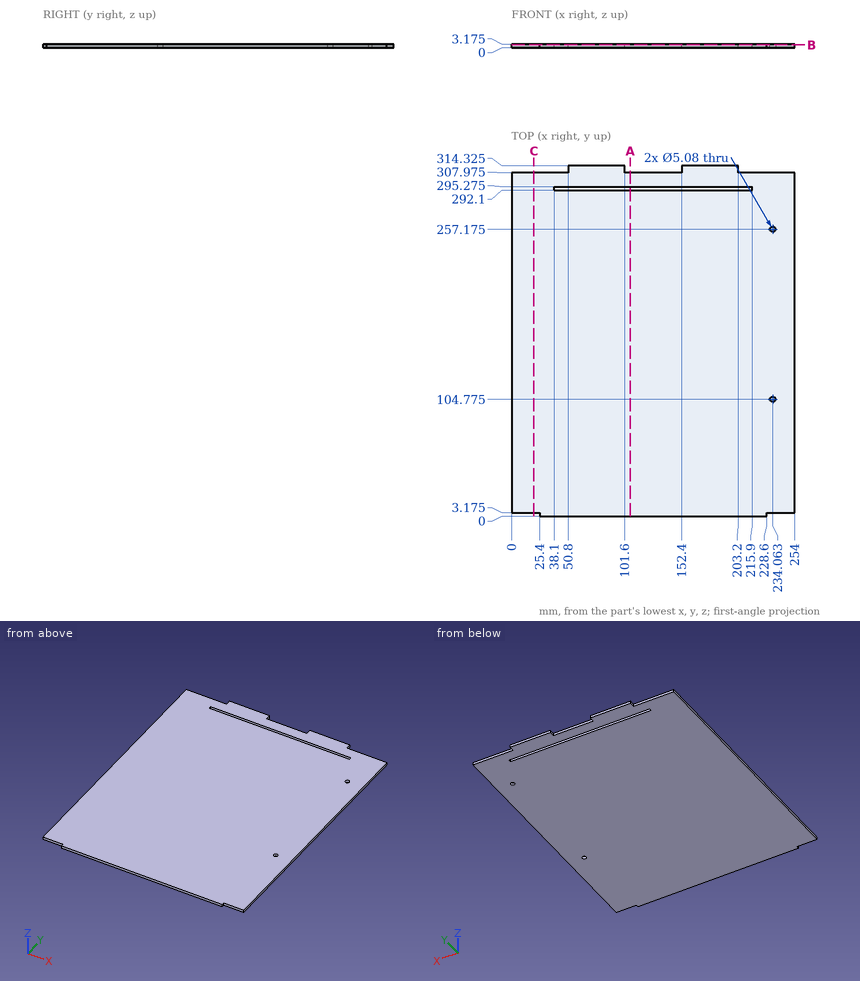
Verification items for this drawing (mm, ordinates from the low corner). Round coordinates to 2 decimals unless told otherwise and drop trailing zeros. Write each loop counter-clockwise with the first axis right and the second up, starting at its lowest first coordinate (ties: lowest second). Pieces come first, ordered by that corner, then holes. Notation, with made-up numbers: (-5.5, 83.5) - (30.5, 83.5) arc R35 cw to (30.5, 116.5) - close; hole circle Ø3 at (8, -10.5). An arc over 180 degrees is marked (long way). Answer as a JSON object with one key per item and string values. Group by question number.
Q1. Go/stop test with flat-tipped pins: pin 1 Ø1 at (y, z) = (294, 1.5) entering from -X; pin 2 Ø4.5 at (x, y) = (234.06, 104.78) entering from -Z; pin 3 Ø1.6 at (y, z) = (310, 1.5) entering from +X; pin 4 Ø1.6 at (x, z) = (246.5, 1.5) entering from -Y (3 decimals). Record where each tip stops, or that it passes through.
Q2. Section check C-C, the plane x = 20. Enter the section's corners in (y, z) (1 decimal).
Q3. Thickness scan on line 1 (Y direction, x = 174.5, z = 1.35) (1 decimal); line 2 (Y direction, x = 102, z = 1.7) (1 decimal); line 3 (Y direction, x = 221.5, z = 0.15) (1 decimal). Record the ranges inside material, lowest first.
Q4. Section check B-B, the plane z = 2.4. Enter the section's corners in (x, y) (1 decimal).
Q5. Section check A-A, the plane x = 106.5. Enter the section's corners in (y, z) (1 decimal).
Found:
{
 "1": {"pin 1": "stops at x = 0", "pin 2": "passes through", "pin 3": "stops at x = 203.2", "pin 4": "stops at y = 3.175"},
 "2": {"outline": "(3.2, 0) - (308, 0) - (308, 3.2) - (3.2, 3.2) - close"},
 "3": {"line 1": "y = 0 to 292.1, 295.3 to 314.3", "line 2": "y = 0 to 292.1, 295.3 to 308", "line 3": "y = 0 to 308"},
 "4": {"outline": "(0, 3.2) - (25.4, 3.2) - (25.4, 0) - (228.6, 0) - (228.6, 3.2) - (254, 3.2) - (254, 308) - (203.2, 308) - (203.2, 314.3) - (152.4, 314.3) - (152.4, 308) - (101.6, 308) - (101.6, 314.3) - (50.8, 314.3) - (50.8, 308) - (0, 308) - close; hole (38.1, 292.1) - (215.9, 292.1) - (215.9, 295.3) - (38.1, 295.3) - close; hole circle Ø5.1 at (234.1, 104.8); hole circle Ø5.1 at (234.1, 257.2)"},
 "5": {"outline": "(0, 0) - (292.1, 0) - (292.1, 3.2) - (0, 3.2) - close; (295.3, 0) - (308, 0) - (308, 3.2) - (295.3, 3.2) - close"}
}
